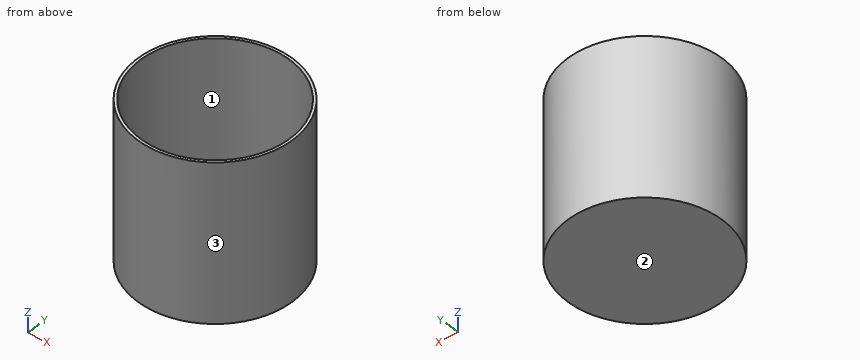
from build123d import *

# Parameters (mm, degrees)
F1_R     = 28.5
F2_DEPTH = 55
F3_D     = 55
F5_R     = 28.5
F6_DEPTH = 3


with BuildPart() as f2:
    # F1 (on Top) → F2 (new body)
    with BuildSketch(Plane.XY):
        Circle(F1_R)
    extrude(amount=F2_DEPTH)

    # F3 (through all)
    with Locations(Plane(origin=(0, 0, 0), x_dir=(1, 0, 0), z_dir=(0, 0, -1))):
        with Locations((0, 0)):
            Hole(F3_D / 2)

    # F5 (on offset) → F6 (join)
    with BuildSketch(Plane.XY.offset(-3)):
        Circle(F5_R)
    extrude(amount=F6_DEPTH)


solid = f2.part
The listing builds one solid part. Answer for the finished solid, in the listing's coordinates (mm). Face numbers are marked on the shaded views. Give positions to 0.01 mm unless a question says otherwise; leave off trailing zeros. Order: outer loops, then holes, each group sorted by start corner. A loop starts at its lowest first (then second) coordinate and runs counter-clockwise, first axis right, second up. Notation, with made-up numbers: (81, 13) -> (88, 13) arc R20 ccw to (88, 22) -> close; hole circle Ø4 at (16.5, 44.5). An arc over 180 degrees is marked (long way). Put each result on its own line as item: value.
Item 1: Straight lines are drawn through the part: line 1 (Y direction, x = 0, z = 22); line 2 (Y direction, x = 14, z = 31.5); line 3 (X direction, y = -14.5, z = 41.5). For each, find the intervals that lie inside material, in ascending order.
Established:
line 1: y = -28.5 to -27.5, 27.5 to 28.5
line 2: y = -24.82 to -23.67, 23.67 to 24.82
line 3: x = -24.54 to -23.37, 23.37 to 24.54
Item 2: A cutting plane is placed at A-A on y = 0. Give the vertices of the cut face in (x, z).
Established:
outline: (-28.5, -3) -> (28.5, -3) -> (28.5, 55) -> (27.5, 55) -> (27.5, 0) -> (-27.5, 0) -> (-27.5, 55) -> (-28.5, 55) -> close
Item 3: A cutting plane is placed at B-B on z = 31.5. Give the vertices of the cut face in (x, y), plus the area to 3 significant figures.
Established:
outline: circle Ø57 at (0, 0); hole circle Ø55 at (0, 0)
area: 176 mm^2
Item 4: Given P1, Ø2, axis at y = 1.5, z = 41, coming from the +X side; P2, Ø3, axis at x = -20.5, z = 43.5, coming from the +Y side; P3, Ø5, axis at x = 10, z = 16.5, coming from the -Y side, each flat-ended and moving along its own axis, determine where each tip first touches the part or whether it passes through.
Established:
P1: stops at x = 28.5
P2: stops at y = 21.24
P3: stops at y = -27.5
Item 5: For a pull along Y with two mould halves and no side action, classify the marked faces 1, 2 and 3 as released by +Y, released by -Y, zero draft, split by the parting line, or undercut.
Established:
face 1: undercut
face 2: zero draft
face 3: split by the parting line
